Design review of the part built by this model. Coordinates are the model's own, in mm. A direction names the side the tool comes from. Give positions to 0.01 mm unless a question says otherwise; leave off trailing zeros. Loops run counter-clockwise (first coordinate to the right, second up) from the corner with the lowest first, then second, coordinate; pieces in that order, holes last. Notation, with made-up numbers: M 6.25,-34.75 L 41.25,-34.75 A14 cw 41.25,-8.75 Z; hole C 11.25,56.25 d10. An arc over 180 degrees is marked long. Use a Markdown table: item, result. Add a question column.
(1) For probe 1 along X at (y, z) = (0, -3); probe 2 along X at (y, z) = (-3.5, -2); probe 3 along Z at (x, y) = (-5.5, 9.75), list the stretches that pass through material, from the lowest coordinate up.
(2) Add section A-A, the plane z = -3.75. Give the boundary of the cut face in (x, y).
(3) Draft analysis for pull direction X (two halves, no side actions). For faces 1 (the face through (0, 0, -1.248)), 2 (the face through (3, 11, 0)), 3 (the face through (3.298, 10.473, -2.292)), state which applies: pulls with the +X half, pulls with the -X half, needs draft (parallel to the pull), parting line crosses it, or undercut.
(4) Insertion check: pin 1 Ø12 at (x, y) = (0.5, 9.5) entering from +Z; pin 2 Ø1.5 at (x, y) = (9, 10) entering from -Z; pin 3 Ø1.5 at (x, y) = (1, 5) entering from -Z; pin 4 Ø5 at (x, y) = (-0.5, -7.5) entering from -Z. Each pin has a flat end and moves straight along its axis. Give the tip position at first contact, or say it passes through.
(5) For faces 4 (the face through (7.5, 4.78, -5.69)), 5 (the face through (-9, 1, -10)), list the 3-axis set-ups (+Z, -Z, +X, -X, +Y, -Y) from which the entire face can be reached by the end or side of a thin tool; tool diameter is ignored.
```python
from build123d import *


with BuildPart() as f1:
    # F0 (on Right) → F1 (revolve)
    with BuildSketch(Plane.YZ):
        with BuildLine():
            Line((10.98, -4.649603), (10.98, 0))
            Line((10.98, 0), (12.98, 0))
            ThreePointArc((12.98, 0), (6.584993, 1.628545), (0, 2.06))
            Line((0, 2.06), (0, -1.247563))
            Line((0, -1.247563), (8.892437, -1.247563))
            Line((8.892437, -1.247563), (8.892437, -10))
            Line((8.892437, -10), (10.98, -10))
            Line((10.98, -10), (10.98, -5.35))
            Line((10.98, -5.35), (10.98, -4.649603))
        make_face()
        with BuildLine():
            ThreePointArc((10.98, -5.35), (11.330199, -4.999801), (10.98, -4.649603))
            Line((10.98, -4.649603), (10.98, -5.35))
        make_face()
    revolve(axis=Axis((0, 0, 0.406218), (0, 0, -1)))


solid = f1.part
```
Established:
| question | item | result |
|---|---|---|
| 1 | probe 1 | -10.98 to -8.89, 8.89 to 10.98 |
| 1 | probe 2 | -10.41 to -8.17, 8.17 to 10.41 |
| 1 | probe 3 | -5.28 to -4.72, 0 to 0.58 |
| 2 | outline | C 0,0 d21.96; hole C 0,0 d17.78 |
| 3 | face 1 | undercut |
| 3 | face 2 | needs draft |
| 3 | face 3 | parting line crosses it |
| 4 | pin 1 | z = 1.98 |
| 4 | pin 2 | z = 0 |
| 4 | pin 3 | z = -1.25 |
| 4 | pin 4 | z = -10 |
| 5 | face 4 | -Z |
| 5 | face 5 | -Z, +X, -X, +Y, -Y |
